Model file for the job. Use its own axes, mm. Round coordinates to 2 decimals unless told otherwise and drop trailing zeros. Order: outer loops, then holes, each group sorted by start corner. A loop starts at its lowest first (then second) coordinate and runs counter-clockwise, first axis right, second up. Notation, with made-up numbers: (-24.75, 10.25) - (34.25, 10.25) arc R27 ccw to (34.25, 36.25) - close; hole circle Ø6 at (-8, 53.25). An arc over 180 degrees is marked (long way). Use one line per item in the form item = value.
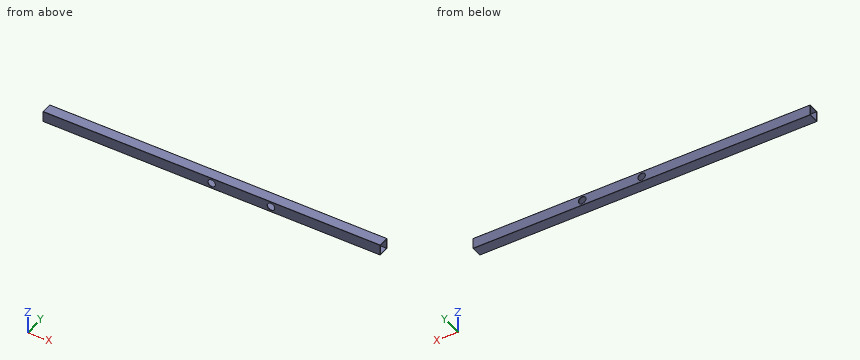
Autodesk Inventor part; units mm, degrees
ref_plane "YZ Plane" through (0, 0, 0) normal (1, 0, 0) x (0, 1, 0)
ref_plane "XZ Plane" through (0, 0, 0) normal (0, 1, 0) x (-1, 0, 0)
ref_plane "XY Plane" through (0, 0, 0) normal (0, 0, 1) x (1, 0, 0)
sketch "Skizze1" plane through (0, 0, 0) normal (1, 0, 0) x (0, 1, 0)
  line L0 (-19, 20) -> (19, 20)
  line L1 (20, 19) -> (20, -19)
  line L2 (19, -20) -> (-19, -20)
  line L3 (-20, -19) -> (-20, 19)
  line L4 (-20, 20) -> (20, -20) construction
  line L5 (20, 20) -> (-20, -20) construction
  line L6 (-17.5, 18) -> (17.5, 18)
  line L7 (18, 17.5) -> (18, -17.5)
  line L8 (17.5, -18) -> (-17.5, -18)
  line L9 (-18, -17.5) -> (-18, 17.5)
  line L10 (-18, 18) -> (18, -18) construction
  line L11 (18, 18) -> (-18, -18) construction
  arc A0 (20, 19) -> (19, 20) centre (19, 19) ccw
  arc A1 (-19, 20) -> (-20, 19) centre (-19, 19) ccw
  arc A2 (-20, -19) -> (-19, -20) centre (-19, -19) ccw
  arc A3 (19, -20) -> (20, -19) centre (19, -19) ccw
  arc A4 (18, 17.5) -> (17.5, 18) centre (17.5, 17.5) ccw
  arc A5 (-17.5, 18) -> (-18, 17.5) centre (-17.5, 17.5) ccw
  arc A6 (-18, -17.5) -> (-17.5, -18) centre (-17.5, -17.5) ccw
  arc A7 (17.5, -18) -> (18, -17.5) centre (17.5, -17.5) ccw
  point P0 (0, 0)
  dimension "d0" = 40
  dimension "d1" = 40
  dimension "d2" = 36
  dimension "d3" = 36
  dimension "d4" = 1
  dimension "d5" = 0.5
extrude "Extrusion1" add sketch "Skizze1" along normal blind 1250
sketch "Skizze2" plane through (0, 20, 19) normal (0, 1, 0) x (1, 0, 0)
  line L0 (0, 19) -> (425, 19)
  line L1 (425, 19) -> (845, 19)
  circle A0 centre (845, 19) radius 14
  line L2 (0, 19) -> (635, 19)
  line L3 (0, 19) -> (625, 19)
  circle A1 centre (625, 19) radius 14
  dimension "d8" = 425
  dimension "d10" = 420
  dimension "d11" = 28
  dimension "d15" = 28
extrude "Extrusion2" cut sketch "Skizze2" against normal through all
properties part number "richtungstange" material "Aluminium 6061"
(1) Slice it at C-C on y = 3.5. Give the cut face in (x, z).
Report:
outline = (0, -20) - (1250, -20) - (1250, -18) - (0, -18) - close; (0, 18) - (1250, 18) - (1250, 20) - (0, 20) - close
(2) Slice it at B-B on x = 301. Give the cut face in (y, z).
Report:
outline = (-20, -19) arc R1 ccw to (-19, -20) - (19, -20) arc R1 ccw to (20, -19) - (20, 19) arc R1 ccw to (19, 20) - (-19, 20) arc R1 ccw to (-20, 19) - close; hole (-18, -17.5) arc R0.5 ccw to (-17.5, -18) - (17.5, -18) arc R0.5 ccw to (18, -17.5) - (18, 17.5) arc R0.5 ccw to (17.5, 18) - (-17.5, 18) arc R0.5 ccw to (-18, 17.5) - close
(3) Slice it at D-D on x = 625. Give the cut face in (y, z), then the cut area to 3 significant figures.
Report:
outline = (-20, -19) arc R1 ccw to (-19, -20) - (19, -20) arc R1 ccw to (20, -19) - (20, -14) - (18, -14) - (18, -17.5) arc R0.5 cw to (17.5, -18) - (-17.5, -18) arc R0.5 cw to (-18, -17.5) - (-18, -14) - (-20, -14) - close; (-20, 14) - (-18, 14) - (-18, 17.5) arc R0.5 cw to (-17.5, 18) - (17.5, 18) arc R0.5 cw to (18, 17.5) - (18, 14) - (20, 14) - (20, 19) arc R1 ccw to (19, 20) - (-19, 20) arc R1 ccw to (-20, 19) - close
area = 191 mm2
(4) Probe probe 1 along X at (y, z) = (-18.9, 0); probe 2 along Z at (x, y) = (491, 14). List the from-to ranges inside material, lowest first. Write a range as [from, to].
Report:
probe_1 = [0, 611], [639, 831], [859, 1250]
probe_2 = [-20, -18], [18, 20]
(5) Slice it at A-A on z = 0. Give the cut face in (x, y).
Report:
outline = (0, -20) - (611, -20) - (611, -18) - (0, -18) - close; (0, 18) - (611, 18) - (611, 20) - (0, 20) - close; (639, -20) - (831, -20) - (831, -18) - (639, -18) - close; (639, 18) - (831, 18) - (831, 20) - (639, 20) - close; (859, -20) - (1250, -20) - (1250, -18) - (859, -18) - close; (859, 18) - (1250, 18) - (1250, 20) - (859, 20) - close
